Check sheet for the modelled part. Datum: model origin and axes. Units: mm. A direction names the side the tool comes from. Round coordinates to 2 decimals unless told otherwise and drop trailing zeros. Write each loop counter-clockwise with the first axis right and the second up, starting at its lowest first coordinate (ties: lowest second). Pieces come first, ordered by that corner, then holes. Notation, with made-up numbers: (48, 67) -> (76, 67) arc R22 cw to (76, 74) -> close; hole circle Ø7 at (-36.75, 74). An arc over 180 degrees is marked (long way). Answer as a JSON object with one key per item and string values. Group by question number.
Autodesk Inventor part; units mm, degrees
ref_plane "YZ Plane" through (0, 0, 0) normal (1, 0, 0) x (0, 1, 0)
ref_plane "XZ Plane" through (0, 0, 0) normal (0, 1, 0) x (-1, 0, 0)
ref_plane "XY Plane" through (0, 0, 0) normal (0, 0, 1) x (1, 0, 0)
sketch "Sketch6" plane through (0, 0, 0) normal (0, 0, 1) x (1, 0, 0)
  line L0 (18, 18) -> (-18, 18)
  line L1 (-18, 18) -> (-18, -18)
  line L2 (-18, -18) -> (18, -18)
  line L3 (18, -18) -> (18, 18)
  line L4 (18, 18) -> (-18, -18) construction
  circle A0 centre (0, -40) radius 5.05
  circle A1 centre (35, 20) radius 5.05
  circle A2 centre (-35, 20) radius 5.05
  line L5 (35, 20) -> (-35, 20) construction
  line L6 (-35, 20) -> (0, -40) construction
  line L7 (0, -40) -> (35, 20) construction
  line L8 (0, 18) -> (0, -18) construction
  line L9 (-47.5046, 28) -> (47.5046, 28)
  line L10 (-18, 18) -> (23.6569, -23.6569) construction
  line L11 (18, 18) -> (-23.6569, -23.6569) construction
  line L12 (47.5046, 28) -> (23.6569, -23.6569)
  line L13 (23.6569, -23.6569) -> (0, -52.6557)
  line L14 (0, -52.6557) -> (-23.6569, -23.6569)
  line L15 (-47.5046, 28) -> (-23.6569, -23.6569)
  line L16 (-35, 20) -> (-42.2633, 16.6468) construction
  line L17 (0, -40) -> (-6.1989, -45.057) construction
  point P0 (0, 0)
  point P1 (0, 0)
  point P2 (60, 0)
  point P3 (0, 28)
  point P4 (0, 0)
  dimension "d30" = 36
  dimension "d31" = 36
  dimension "d33" = 10.1
  dimension "d37" = 69.4622
  dimension "d52" = 70
  dimension "d53" = 8
  dimension "d54" = 20
  dimension "d57" = 8
  dimension "d59" = 8
  dimension "d60" = 95.0092
  dimension "d61" = 60
  dimension "d62" = 8
  dimension "d63" = 8
extrude "Plate3" add sketch "Sketch6" along normal blind 3
fillet "Corner Round2" radius 6 5 edges at (-47.5046, 28, 1.5) (47.5046, 28, 1.5) (0, -52.6557, 1.5) (-23.6569, -23.6569, 1.5) (23.6569, -23.6569, 1.5)
equation "\"d41\" = Thickness"
equation "\"BendReliefWidth\" = Thickness"
equation "\"BendReliefDepth\" = 0.5 * Thickness"
equation "\"CornerReliefSize\" = 4 * Thickness"
equation "\"MinimumRemnant\" = 2 * Thickness"
equation "\"TransitionRadius\" = BendRadius"
equation "\"JacobiRadiusSize\" = BendRadius"
equation "\"GapSize\" = Thickness"
properties part number "MNT-CDF-504 small tube flange" material "Stainless Steel"
(1) Go/stop test with flat-tipped pins: pin 1 Ø9 at (x, y) = (-35, 20) entering from +Z; pin 2 Ø0.9 at (y, z) = (-6, 2) entering from -X; pin 3 Ø0.9 at (y, z) = (-7, 1.5) entering from +X; pin 4 Ø1.5 at (y, z) = (-10, 0.5) entering from +X. Record where each tip stops, or that it passes through.
(2) Access from +Z, -Z, +X, -X, +Y, -Y to the whole of each face (thin tool, end or side, straight path). Record for faces 1 (the flat face through (-18, 0, 1)), 2 (the flat face through (-1, -19, 0)).
(3) Section check C-C on y = -0.5. Record the cut outline in (x, z), then the cut area to 3 significant figures.
(4) Release check for a two-part mould opening along X. For faces 3 (the flat face through (-33.912, -1.444, 1.479)), 4 (the flat face through (-1, -19, 3)), 5 (the cylindrical face through (-40.045, 19.778, 1.479)) record: pulls with the +X half, pulls with the -X half, needs draft (parallel to the pull), parting line crosses it, or undercut.
(5) Section check D-D on y = 22. Record the cut outline in (x, z), then the cut area to 3 significant figures.
(6) Scan lines: line 1 along Y through (x, z) = (0, 2); line 2 along Y through (x, z) = (-3, 2.2); line 3 along X through (y, z) = (9.5, 2.55). Record each from-to range of solid material in increasing order.
(7) Section check A-A on z = 1.1. Record the cut outline in (x, y).
(8) Section check B-B on x = 0. Record the cut outline in (y, z), then the cut area to 3 significant figures.
Data:
{
 "1": {"pin 1": "passes through", "pin 2": "stops at x = -32.02", "pin 3": "stops at x = 31.55", "pin 4": "stops at x = 30.31"},
 "2": {"face 1": "+Z, -Z", "face 2": "-Z, +X, -X, +Y, -Y"},
 "3": {"outline": "(-34.35, 0) -> (-18, 0) -> (-18, 3) -> (-34.35, 3) -> close; (18, 0) -> (34.35, 0) -> (34.35, 3) -> (18, 3) -> close", "area": "98.1 mm²"},
 "4": {"face 3": "pulls with the -X half", "face 4": "needs draft", "face 5": "undercut"},
 "5": {"outline": "(-44.13, 0) -> (-39.64, 0) -> (-39.64, 3) -> (-44.13, 3) -> close; (-30.36, 0) -> (30.36, 0) -> (30.36, 3) -> (-30.36, 3) -> close; (39.64, 0) -> (44.13, 0) -> (44.13, 3) -> (39.64, 3) -> close", "area": "209 mm²"},
 "6": {"line 1": "y = -49.16 to -45.05, -34.95 to -18, 18 to 28", "line 2": "y = -48.36 to -44.06, -35.94 to -18, 18 to 28", "line 3": "x = -38.96 to -18, 18 to 38.96"},
 "7": {"outline": "(-43.57, 19.49) -> (-23.98, -22.97) arc R6 ccw to (-23.18, -24.25) -> (-4.65, -46.96) arc R6 ccw to (4.65, -46.96) -> (23.18, -24.25) arc R6 ccw to (23.98, -22.97) -> (43.57, 19.49) arc R6 ccw to (38.13, 28) -> (-38.13, 28) arc R6 ccw to start; hole circle Ø10.1 at (-35, 20); hole (-18, -18) -> (18, -18) -> (18, 18) -> (-18, 18) -> close; hole circle Ø10.1 at (0, -40); hole circle Ø10.1 at (35, 20)"},
 "8": {"outline": "(-49.16, 0) -> (-45.05, 0) -> (-45.05, 3) -> (-49.16, 3) -> close; (-34.95, 0) -> (-18, 0) -> (-18, 3) -> (-34.95, 3) -> close; (18, 0) -> (28, 0) -> (28, 3) -> (18, 3) -> close", "area": "93.2 mm²"}
}
